Part model, mm, in its own coordinate system. A direction names the side the tool comes from. Round coordinates to 2 decimals unless told otherwise and drop trailing zeros. Loops run counter-clockwise (first coordinate to the right, second up) from the corner with the lowest first, then second, coordinate; pieces in that order, holes last. Notation, with made-up numbers: (75.25, 51.25) -> (89.25, 51.25) arc R33 ccw to (89.25, 83.25) -> close; hole circle Ø4 at (24, 85). An arc over 180 degrees is marked (long way). Answer as CSV lines item,"result".
from build123d import *

# Parameters (mm, degrees)
F0_R     = 3
F1_DEPTH = 6.8
F2_R     = 6.125
F3_DEPTH = 3.9
F4_SIZE  = 0.5
F5_R     = 4.15
F6_DEPTH = 4.02


with BuildPart() as f1:
    # F0 (on Top) → F1 (new body)
    with BuildSketch(Plane.XY):
        Circle(F0_R)
    extrude(amount=F1_DEPTH)

    # F2 (on face) → F3 (join)
    with BuildSketch(Plane(origin=(0, 0, 0), x_dir=(1, 0, 0), z_dir=(0, 0, -1))):
        Circle(F2_R)
    extrude(amount=F3_DEPTH)

    # F4
    f4_edges = [f1.edges().sort_by_distance(p)[0] for p in [
        (-6.125, 0, 0),
        (-6.125, 0, -3.9),
    ]]
    chamfer(f4_edges, length=F4_SIZE)

    # F5 (on face) → F6 (join)
    with BuildSketch(Plane.XY.offset(6.8)):
        Circle(F5_R)
    extrude(amount=-F6_DEPTH)


solid = f1.part
Q1. Drill centre lines: line 1 along Z through (x, y) = (1.25, -3.75); line 2 along Z through (x, y) = (4.25, -0.75); line 3 along Y through (x, z) = (-0.75, -1.75). Where is each one in solid material? Low to high.
Geometry results:
line 1,"-3.9 to 0, 2.78 to 6.8"
line 2,"-3.9 to 0"
line 3,"-6.08 to 6.08"
Q2. Saw through at A-A, the plane x = 0. Write the cut outline in (y, z) (3 decimals).
Geometry results:
outline,"(-6.125, -3.4) -> (-5.625, -3.9) -> (5.625, -3.9) -> (6.125, -3.4) -> (6.125, -0.5) -> (5.625, 0) -> (3, 0) -> (3, 2.78) -> (4.15, 2.78) -> (4.15, 6.8) -> (-4.15, 6.8) -> (-4.15, 2.78) -> (-3, 2.78) -> (-3, 0) -> (-5.625, 0) -> (-6.125, -0.5) -> close"
Q3. Saw through at C-C, the plane z = 1.25. Write the cut outline in (x, y), then the cut area to 3 significant figures.
Geometry results:
outline,"circle Ø6 at (0, 0)"
area,"28.3 mm2"
Q4. Drop flat-ended pins along their axis: P1, Ø1.5, axis at x = 1, z = -0.5, coming from the +Y side; P2, Ø3, axis at x = -2.5, z = 3, coming from the -Y side; P3, Ø1, axis at y = 2, z = 5.5, coming from the +X side. Give the stop position or say it passes through.
Geometry results:
P1,"y = 6.12"
P2,"y = -4.03"
P3,"x = 3.87"
Q5. Saw through at D-D, the plane z = -2. Write the cut outline in (x, y) (3 decimals), then the cut area to 3 significant figures.
Geometry results:
outline,"circle Ø12.25 at (0, 0)"
area,"118 mm2"
Q6. Which spindle directions (+Z, -Z, +X, -X, +Y, -Y) get a long thin tool onto all of the face, cutting with end or side? Do faces 1 (the face through (2.4, 2.4, 0)), 2 (the face through (-0.9, -4.05, 4.82)), 3 (the face through (0, 0, -3.9)). Say none if no direction does.
Geometry results:
face 1,"none"
face 2,"+Z"
face 3,"-Z, +X, -X, +Y, -Y"
Q7. Two-plate mould, pull along Z, no slides. Class faces 4 (the face through (-3, 0, 1)), 5 (the face through (0, 0, 6.8)), 6 (the face through (3.293, -5.165, -1.93)): pulls with the +Z half, pulls with the -Z half, needs draft (parallel to the pull), parting line crosses it, or undercut.
Geometry results:
face 4,"undercut"
face 5,"pulls with the +Z half"
face 6,"needs draft"
